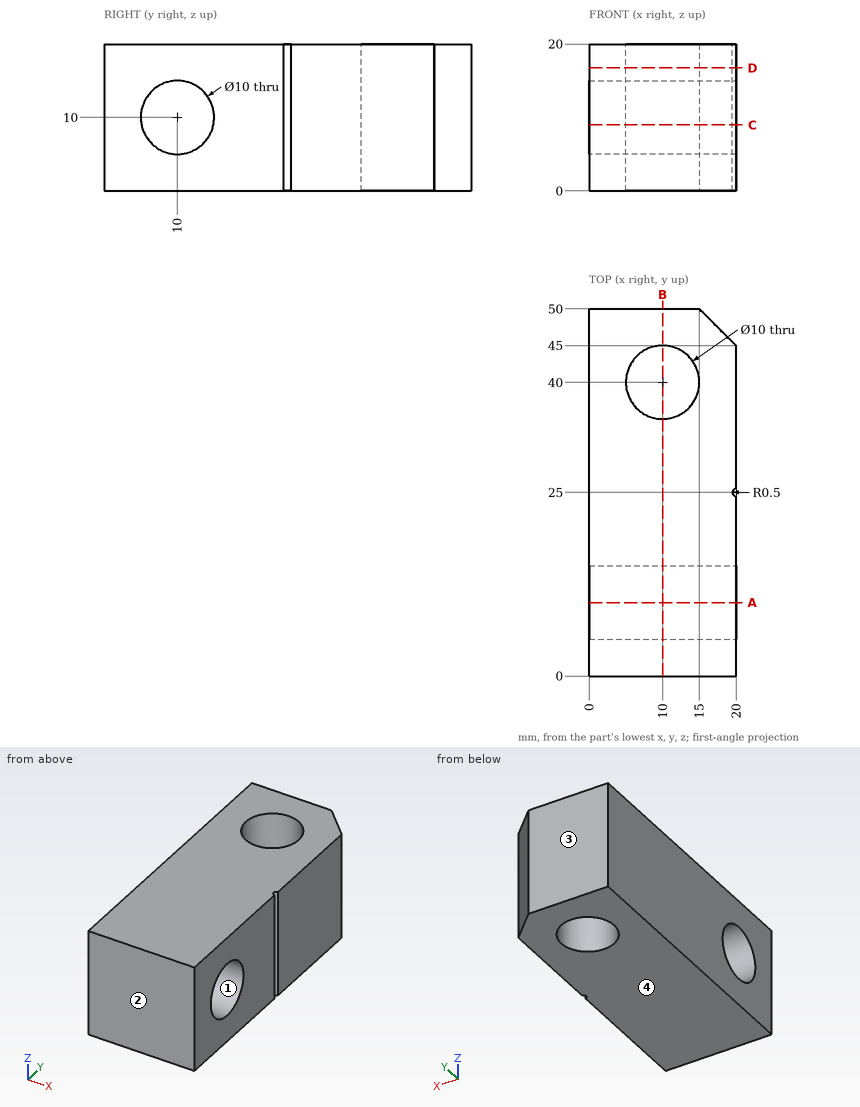
Input: dimensioned drawing with shaded views. Units: mm. Origin: part minimum x, y, z. Give positions to 0.01 mm unless a question says otherwise; leave off trailing zeros. Write each loop counter-clockwise with the first axis right and the second up, starting at its lowest first coordinate (ties: lowest second). Pieces come first, ordered by that corner, then holes. Notation, with made-up numbers: (-7, 43.5) -> (49, 43.5) arc R17 cw to (49, 74.5) -> close; hole circle Ø8 at (43, 14). An arc over 180 degrees is marked (long way). Answer as a JSON object with one key per item and string values.
1. Mould query, pull axis Y, two halves, no side actions, for the marked faces 1, 2, 3 and 4. Classes: pulls with the +Y half, pulls with the -Y half, needs draft (parallel to the pull), parting line crosses it, or undercut.
Ans:
{"face 1": "undercut", "face 2": "pulls with the -Y half", "face 3": "pulls with the +Y half", "face 4": "needs draft"}
2. Cut plane A-A on y = 10. Output: boundary loops of the cut face in (x, z), and give its area (3 significant figures).
Ans:
{"outline": "(0, 0) -> (20, 0) -> (20, 5) -> (0, 5) -> close; (0, 15) -> (20, 15) -> (20, 20) -> (0, 20) -> close", "area": "200 mm^2"}
3. Ray query, probe 1 along Y at (x, z) = (9.75, 10); probe 2 along Y at (x, z) = (10, 5.75); probe 3 along X at (y, z) = (35.5, 15.25). Return the intervals inside material, ascending. Write a range as from..to.
Ans:
{"probe 1": "y = 0..5, 15..35.01, 44.99..50", "probe 2": "y = 0..7.37, 12.63..35, 45..50", "probe 3": "x = 0..7.82, 12.18..20"}
4. Cut plane B-B on x = 10. Output: boundary loops of the cut face in (y, z), and give its area (3 significant figures).
Ans:
{"outline": "(0, 0) -> (35, 0) -> (35, 20) -> (0, 20) -> close; (45, 0) -> (50, 0) -> (50, 20) -> (45, 20) -> close; hole circle Ø10 at (10, 10)", "area": "721 mm^2"}
5. Cut plane D-D on z = 16.75. Output: boundary loops of the cut face in (x, y), and give its area (3 significant figures).
Ans:
{"outline": "(0, 0) -> (20, 0) -> (20, 24.5) arc R0.5 cw to (20, 25.5) -> (20, 45) -> (15, 50) -> (0, 50) -> close; hole circle Ø10 at (10, 40)", "area": "909 mm^2"}
6. Cut plane C-C on z = 9. Output: boundary loops of the cut face in (x, y), and give its area (3 significant figures).
Ans:
{"outline": "(0, 0) -> (20, 0) -> (20, 5.1) -> (0, 5.1) -> close; (0, 14.9) -> (20, 14.9) -> (20, 24.5) arc R0.5 cw to (20, 25.5) -> (20, 45) -> (15, 50) -> (0, 50) -> close; hole circle Ø10 at (10, 40)", "area": "713 mm^2"}
